Can you work these out from the model? Positions are in its coordinate system, mm. A direction names the side the tool comes from. Give positions to 0.01 mm unless a question says otherwise; leave off trailing zeros. Order: outer loops, then holes, each group sorted by start corner. A loop starts at its lowest first (then second) coordinate and runs counter-clockwise, first axis right, second up. Notation, with made-up numbers: (-32.75, 55.25) -> (23.25, 55.25) arc R28 cw to (23.25, 92.25) -> close; hole circle Ø1 at (83.25, 78). An arc over 180 degrees is marked (long way). Answer as a JSON object with one key per item and string values.
```python
from build123d import *

# Parameters (mm, degrees)
SKETCH1_W           = 43.16
SKETCH1_H           = 72
BOSS_EXTRUDE1_DEPTH = 9
SKETCH2_W           = 37.08
SKETCH2_H           = 4
CUT_EXTRUDE1_DEPTH  = 73
SKETCH3_W           = 28.08
SKETCH3_H           = 7.5
CUT_EXTRUDE2_DEPTH  = 6
SKETCH4_W           = 16.08
SKETCH4_H           = 64.5
BOSS_EXTRUDE2_DEPTH = 4
SKETCH5_W           = 16.08
SKETCH5_H           = 9
BOSS_EXTRUDE3_DEPTH = 7.5
SKETCH6_W           = 4
SKETCH6_H           = 4
CUT_EXTRUDE3_DEPTH  = 73
BOSS_EXTRUDE4_DEPTH = 4
SCALE1_SCALE        = 0.25


with BuildPart() as part:
    # Sketch1 → Boss-Extrude1 (new body)
    with BuildSketch(Plane(origin=(0, 0, 0), x_dir=(-1, 0, 0), z_dir=(0, 0, -1))):
        Rectangle(SKETCH1_W, SKETCH1_H)
    extrude(amount=-BOSS_EXTRUDE1_DEPTH)

    # Sketch2 → Cut-Extrude1 (cut, through all)
    with BuildSketch(Plane(origin=(0, 36, 0), x_dir=(-1, 0, 0), z_dir=(0, 1, 0))):
        with Locations((-3.04, 7)):
            Rectangle(SKETCH2_W, SKETCH2_H)
    extrude(amount=-CUT_EXTRUDE1_DEPTH, mode=Mode.SUBTRACT)

    # Sketch3 → Cut-Extrude2 (cut, through all)
    with BuildSketch(Plane.XY.offset(5)):
        with Locations((7.54, -32.25)):
            Rectangle(SKETCH3_W, SKETCH3_H)
    extrude(amount=-CUT_EXTRUDE2_DEPTH, mode=Mode.SUBTRACT)

    # Sketch4 → Boss-Extrude2 (add)
    with BuildSketch(Plane.XY.offset(5)):
        with Locations((13.54, 3.75)):
            Rectangle(SKETCH4_W, SKETCH4_H)
    extrude(amount=BOSS_EXTRUDE2_DEPTH)

    # Sketch5 → Boss-Extrude3 (add)
    with BuildSketch(Plane.XZ.offset(28.5)):
        with Locations((13.54, 4.5)):
            Rectangle(SKETCH5_W, SKETCH5_H)
    extrude(amount=BOSS_EXTRUDE3_DEPTH)

    # Sketch6 → Cut-Extrude3 (cut, through all)
    with BuildSketch(Plane(origin=(0, 36, 0), x_dir=(-1, 0, 0), z_dir=(0, 1, 0))):
        with Locations((-10.5, 7)):
            Rectangle(SKETCH6_W, SKETCH6_H)
    extrude(amount=-CUT_EXTRUDE3_DEPTH, mode=Mode.SUBTRACT)

    # Sketch7 → Boss-Extrude4 (add)
    with BuildSketch(Plane.XY.offset(5)):
        Polygon((-2.5, -1), (4.5, -1), (4.5, -14), (0.5, -21), (-2.5, -21), align=None)
    extrude(amount=BOSS_EXTRUDE4_DEPTH)


with BuildPart() as part_1:
    # Scale1: scaled about (0.900583751, 0.451348466, 3.739254469)
    add(part.part.scale(SCALE1_SCALE).moved(Location((0.675437813, 0.33851135, 2.804440852))))


solid = part_1.part
```
1. If we section it at C-C on x = -3: Please give me the cut outline in (y, z).
Worked answers:
{"outline": "(-8.66, 2.8) -> (9.34, 2.8) -> (9.34, 4.05) -> (-8.66, 4.05) -> close"}
2. If we section it at B-B on y = -0.25: Please give me the cut outline in (x, z).
Worked answers:
{"outline": "(-4.72, 2.8) -> (6.07, 2.8) -> (6.07, 5.05) -> (3.8, 5.05) -> (3.8, 4.05) -> (2.8, 4.05) -> (2.8, 5.05) -> (2.05, 5.05) -> (2.05, 4.05) -> (1.8, 4.05) -> (1.8, 5.05) -> (0.05, 5.05) -> (0.05, 4.05) -> (-3.2, 4.05) -> (-3.2, 5.05) -> (-4.72, 5.05) -> close"}
3. If we mould it in two halves opening along X, with no side actions, what happens to faces 1 (the face through (6.07, 0, 4)), 2 (the face through (5, 0, 5.054)), 3 (the face through (1.8, -1.5, 4.5))? For each: +X half, -X half, draft (parallel to the pull), parting line (faces both ways), or undercut.
Worked answers:
{"face 1": "+X half", "face 2": "draft", "face 3": "undercut"}
4. If we section it at D-D on z = 3.1: Please give me the cut outline in (x, y).
Worked answers:
{"outline": "(-4.72, -8.66) -> (-0.95, -8.66) -> (-0.95, -6.79) -> (2.05, -6.79) -> (2.05, -8.66) -> (6.07, -8.66) -> (6.07, 9.34) -> (-4.72, 9.34) -> close"}
5. For faces 4 (the face through (-0.95, -8, 3)), 5 (the face through (2.05, 0.5, 4.4)), 6 (the face through (3.8, 0.5, 4.5)), which set-ups out of +Z, -Z, +X, -X, +Y, -Y let a thin tool reach every point of the face, with its end or its side?
Worked answers:
{"face 4": "+Z, -Z, -Y", "face 5": "+Z, -Y", "face 6": "+Z, +Y, -Y"}
6. If we section it at A-A on z = 4.8: Please give me the cut outline in (x, y), then the cut area to 3 significant figures.
Worked answers:
{"outline": "(-4.72, -8.66) -> (-3.2, -8.66) -> (-3.2, 9.34) -> (-4.72, 9.34) -> close; (0.05, -4.91) -> (0.8, -4.91) -> (1.8, -3.16) -> (1.8, 0.09) -> (0.05, 0.09) -> close; (2.05, -8.66) -> (2.8, -8.66) -> (2.8, 9.34) -> (2.05, 9.34) -> close; (3.8, -8.66) -> (6.07, -8.66) -> (6.07, 9.34) -> (3.8, 9.34) -> close", "area": "89.6 mm²"}
7. Please list where these lines run through material, in increasing order: L1, parallel to X at y = 6.5, z = 4.65; L2, parallel to X at y = -0.25, z = 4.15; L3, parallel to Z at x = -1.5, y = 6.25.
Worked answers:
{"L1": "-4.72 to -3.2, 2.05 to 2.8, 3.8 to 6.07", "L2": "-4.72 to -3.2, 0.05 to 1.8, 2.05 to 2.8, 3.8 to 6.07", "L3": "2.8 to 4.05"}
